Design review of the part built by this model. Coordinates are the model's own, in mm. Give positions to 0.01 mm unless a question says otherwise; leave off trailing zeros. Write each loop counter-clockwise with the first axis right and the second up, starting at its lowest first coordinate (ties: lowest second). Pieces come first, ordered by that corner, then holes. Notation, with made-up numbers: M 58.25,-31.5 L 85.25,-31.5 A26 ccw 85.25,-14.5 Z; hole C 64,41.5 d10. An arc over 180 degrees is marked long. Use a Markdown table: item, result. Add a question column.
```python
from build123d import *

# Parameters (mm, degrees)
F1_DEPTH = 2.6


with BuildPart() as f1:
    # F0 (on Top) → F1 (new body)
    with BuildSketch(Plane.XY):
        with BuildLine():
            ThreePointArc((31.762156, -1.999012), (29.825, 0), (31.762156, 1.999012))
            ThreePointArc((31.762156, 1.999012), (0, 31.825), (-31.762156, 1.999012))
            ThreePointArc((-31.762156, 1.999012), (-30.38874, 1.391818), (-29.825, 0))
            ThreePointArc((-29.825, 0), (-30.38874, -1.391818), (-31.762156, -1.999012))
            ThreePointArc((-31.762156, -1.999012), (-22.236949, -22.767273), (-1.25, -31.800442))
            Line((-1.25, -31.800442), (-1.25, 10.825))
            Line((-1.25, 10.825), (1.25, 10.825))
            Line((1.25, 10.825), (1.25, -31.800442))
            ThreePointArc((1.25, -31.800442), (22.236949, -22.767273), (31.762156, -1.999012))
        make_face()
    extrude(amount=F1_DEPTH)


solid = f1.part
```
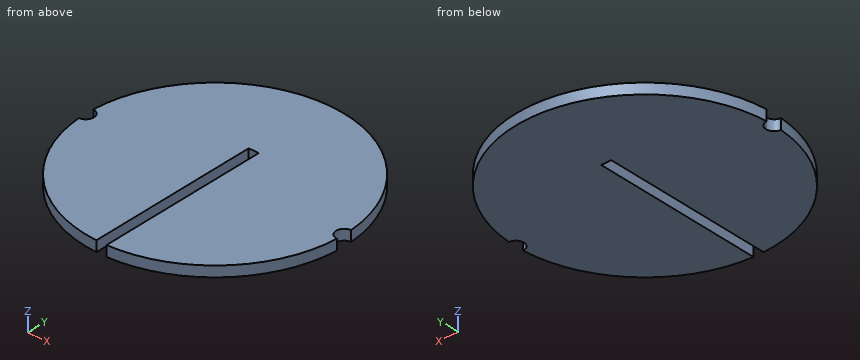
(1) Add section D-D on x = 0. Give the boundary of the cut face in (y, z) (3 decimals).
(2) Add section A-A on y = -21.5. Give the boundary of the cut face in (x, z).
(3) Add section B-B on z = 0.55. Give the boundary of the cut face in (x, y) (3 decimals).
(4) Add section C-C on y = -1. Give the boundary of the cut face in (x, z).
(5) For pin 1 (0.8 mm diameter, centred on y = -3, z = 0.5, fed in from +X); pin 2 (1.5 mm diameter, centred on x = 9, z = 2.5, fed in from -Y); pin 3 (0.8 mm diameter, centred on y = -15, z = 1, fed in from -X), all flat-tipped, find the tip position at first contact; note any pin that passes through.
(6) Wall thickness on L1, parallel to X at y = 1, z = 2.1; L2, parallel to X at y = 3, z = 1.2; L3, parallel to Y at x = 0.5, z = 0.55 (3 decimals): over which ranges is each line inside the solid? List them lowest first.
From the geometry:
| question | item | result |
|---|---|---|
| 1 | outline | M 10.825,0 L 31.825,0 L 31.825,2.6 L 10.825,2.6 Z |
| 2 | outline | M -23.46,0 L -1.25,0 L -1.25,2.6 L -23.46,2.6 Z; M 1.25,0 L 23.46,0 L 23.46,2.6 L 1.25,2.6 Z |
| 3 | outline | M -31.762,-1.999 A31.825 ccw -1.25,-31.8 L -1.25,10.825 L 1.25,10.825 L 1.25,-31.8 A31.825 ccw 31.762,-1.999 A2 cw 31.762,1.999 A31.825 ccw -31.762,1.999 A2 cw Z |
| 4 | outline | M -30.09,0 L -1.25,0 L -1.25,2.6 L -30.09,2.6 Z; M 1.25,0 L 30.09,0 L 30.09,2.6 L 1.25,2.6 Z |
| 5 | pin 1 | stops at x = 31.72 |
| 5 | pin 2 | stops at y = -30.74 |
| 5 | pin 3 | stops at x = -28.28 |
| 6 | L1 | x = -30.09 to -1.25, 1.25 to 30.09 |
| 6 | L2 | x = -31.68 to -1.25, 1.25 to 31.68 |
| 6 | L3 | y = 10.825 to 31.821 |
